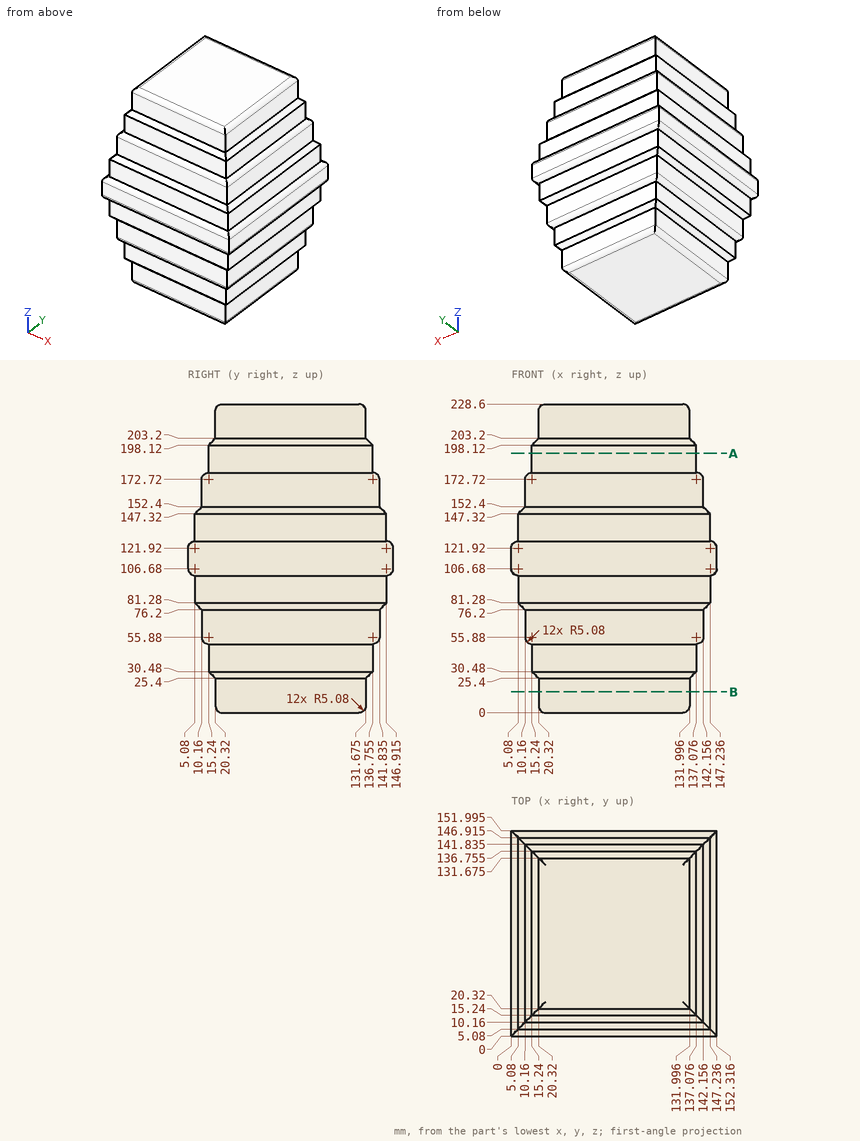
Check sheet for the drawn part. Datum: minimum x, y, z corner. Units: mm. Give positions to 0.01 mm unless a question says otherwise; leave off trailing zeros. Loops run counter-clockwise (first coordinate to the right, second up) from the corner with the lowest first, then second, coordinate; pieces in that order, holes last. Notation, with made-up numbers: M -27.5,18.5 L -11.5,18.5 A7 cw -11.5,28.5 Z; hole C 86,61 d3. An arc over 180 degrees is marked long. Return JSON: item names as keys, results as strings.
1) Section check B-B, the plane z = 15.5. Enter the section's corners in (x, y) (3 decimals).
Findings:
{"outline": "M 20.32,20.32 L 131.996,20.32 L 131.996,131.675 L 20.32,131.675 Z"}
2) Material ranges on L1, parallel to X at y = 129, z = 196.5; L2, parallel to Y at x = 104, z = 59.5 (3 decimals); L3, parallel to X at y = 84, z = 101, recorded low to high. Write a range as [from, to].
Findings:
{"L1": "x = [15.24, 137.08]", "L2": "y = [10.16, 141.835]", "L3": "x = [5.08, 147.24]"}
3) Section check A-A, the plane z = 192. Enter the section's corners in (x, y) (3 decimals).
Findings:
{"outline": "M 15.24,15.24 L 137.076,15.24 L 137.076,136.755 L 15.24,136.755 Z"}
4) Gauge pin test, flat ends, axial feed: P1, Ø10, axis at x = 73, z = 214, coming from the +Y side (3 decimals); P2, Ø8, axis at x = 90.5, z = 136, coming from the +Y side (3 decimals); P3, Ø6, axis at y = 97, z = 213.5, coming from the -X side. Record the tip position at first contact, or that the pin passes through.
Findings:
{"P1": "stops at y = 131.675", "P2": "stops at y = 146.915", "P3": "stops at x = 20.32"}
